Model file for the job. Use its own axes, mm. Face numbers are marked on the shaded views. Coordinates: 2 decimals unless noted, no trailing zeros. Loops run counter-clockwise (first coordinate to the right, second up) from the corner with the lowest first, then second, coordinate; pieces in that order, holes last.
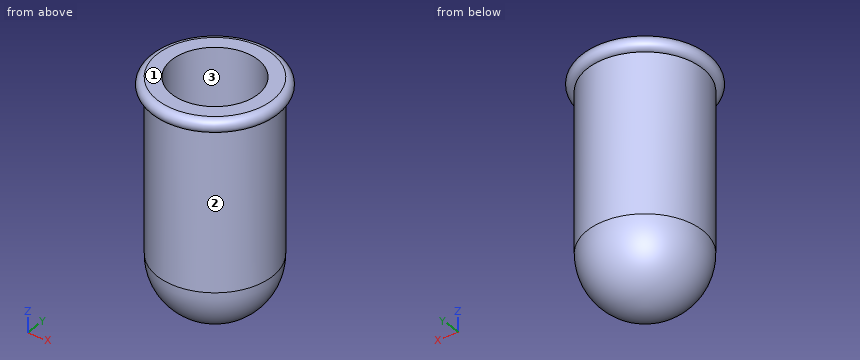
from build123d import *

# Parameters (mm, degrees)
F2_R = 12.7
F3_T = 3.175


# Not quite as in the source:
# - a shell that OpenCascade refuses in one call is made with other operations: the cavity is built on its own and cut out


with BuildPart() as f1:
    # F0 (on Front) → F1 (revolve)
    with BuildSketch(Plane.XZ):
        Polygon((0, 50.8), (0, 0), (12.7, 0), (12.7, 47.6801507175), (12.7, 50.8), align=None)
        with BuildLine():
            ThreePointArc((12.7, 47.6801507175), (14.2599246413, 49.2400753587), (12.7, 50.8))
            Line((12.7, 50.8), (12.7, 47.6801507175))
        make_face()
    revolve(axis=Axis((0, 0, 25.4), (0, 0, 1)))

    # F2
    f2_edges = [f1.edges().sort_by_distance(p)[0] for p in [
        (-12.7, 0, 0),
    ]]
    fillet(f2_edges, radius=F2_R)

    # F3: shell of thickness 3.175, made by hand


with BuildPart() as f3_core1:
    # F3_t2: copy of F1
    add(f1.part)

    # the walls: a layer under each face that stays
    f3_faces = [f3_core1.faces().sort_by_distance(p)[0] for p in [
        (-12.7, 0, 30.1900753587),
        (-8.9802561211, 0, 3.7197438789),
    ]]
    thicken(f3_faces, amount=-F3_T, mode=Mode.SUBTRACT)

    # F3_s3 → F3_t4 (revolve, cut)
    with BuildSketch(Plane.XZ):
        Polygon((12.73175, 47.6484007175), (9.525, 47.6801507175), (9.525, 50.8551507175), (12.7, 50.8551507175), align=None)
    revolve(axis=Axis((0, 0, 47.6801507175), (0, 0, 1)), mode=Mode.SUBTRACT)


with BuildPart() as f1_1:
    add(f1.part)

    # what is left inside the walls is the cavity
    f3_cavity = [f3_core1.part.solids().sort_by_distance(p)[0] for p in [
        (-9.49325, 0, 25.4),
    ]]
    add(f3_cavity, mode=Mode.SUBTRACT)


solid = f1_1.part
Q1. Slice it at C-C (z = 29). List the corners of the cut face in (x, y) (3 decimals), and give its area (3 significant figures).
Answers:
outline: circle Ø25.4 at (0, 0); hole circle Ø19.05 at (0, 0)
area: 222 mm2
Q2. Drill centre lines: line 1 (Y direction, x = 0, z = 36.5) (3 decimals); line 2 (Y direction, x = 2.5, z = 16); line 3 (X direction, y = 2, z = 27). Where is each one in solid material? Low to high.
Answers:
line 1: y = -12.7 to -9.525, 9.525 to 12.7
line 2: y = -12.45 to -9.19, 9.19 to 12.45
line 3: x = -12.54 to -9.31, 9.31 to 12.54
Q3. Mould opens along X. For the marked faces 1, 2 and 3 say: +X half, -X half, draft (parallel to the pull), parting line (faces both ways), or undercut.
Answers:
face 1: draft
face 2: parting line
face 3: undercut
Q4. Slice it at A-A (x = 0). List the corners of the cut face in (y, z) (3 decimals).
Answers:
outline: (-12.7, 12.7) arc R12.7 ccw to (12.7, 12.7) - (12.7, 47.68) arc R1.56 ccw to (12.7, 50.8) - (9.525, 50.8) - (9.525, 12.7) arc R9.525 cw to (-9.525, 12.7) - (-9.525, 50.8) - (-12.7, 50.8) arc R1.56 ccw to (-12.7, 47.68) - close
Q5. Flat gauge pins, fed straight in: P1, Ø8, axis at x = 2, z = 31.5, coming from the +Y side; P2, Ø8, axis at y = -3.5, z = 31.5, coming from the +X side; P3, Ø1, axis at y = -3.5, z = 11, coming from the +X side. Where does each tip first touch, or does it go through?
Answers:
P1: stops at y = 12.7
P2: stops at x = 12.7
P3: stops at x = 12.24
